The listing builds one solid part. Answer for the finished solid, in the listing's coordinates (mm). Face numbers are marked on the shaded views. Give positions to 0.01 mm unless a question says otherwise; leave off trailing zeros. Order: outer loops, then holes, each group sorted by start corner. A loop starts at its lowest first (then second) coordinate and runs counter-clockwise, first axis right, second up. Notation, with made-up numbers: (-12, -9.75) - (6, -9.75) arc R17 ccw to (6, 15.25) - close; hole circle Ø10 at (36.25, -2.5). An arc over 180 degrees is marked (long way). Answer as CSV lines item,"result". Start each with the question number.
1. Section C-C on y = 2.75 is taken. Give the vertices of the cut face in (x, z), and give its area (3 significant figures).
2. A flat-ended cylindrical pin translates along its axis: pin 1 (1.5 mm diameter, centred on x = 16.5, y = 12.5, fed in from -Z). Find the tip coordinate at first contact, or state that the pin passes through.
3. Section B-B on y = 22.5 is taken. Give the vertices of the cut face in (x, z).
4. Consider line 1 along X through (y, z) = (2.25, 8.25); line 2 along Y through (x, z) = (10, 4.75). Determine where each line is inside the solid, lowest interval first. Write a range as [from, to].
5. Determine the mould class of the marked faces 1, 2 and 3 for opening direction X: +X half, -X half, draft (parallel to the pull), parting line (faces both ways), or undercut.
6. Section A-A on z = 8.5 is taken. Give the vertices of the cut face in (x, y), and give its area (3 significant figures).
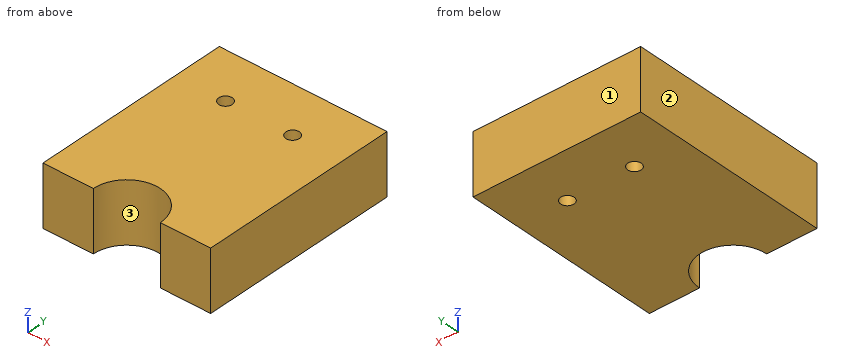
from build123d import *

# Parameters (mm, degrees)
SKETCH1_W           = 25
SKETCH1_H           = 30
BOSS_EXTRUDE1_DEPTH = 9
CUT_EXTRUDE3_DEPTH  = 41.074929819
SKETCH5_R           = 1
CUT_EXTRUDE4_DEPTH  = 41.074929819


with BuildPart() as part:
    # Sketch1 → Boss-Extrude1 (new body)
    with BuildSketch(Plane.XY):
        with Locations((12.5, 15)):
            Rectangle(SKETCH1_W, SKETCH1_H)
    extrude(amount=BOSS_EXTRUDE1_DEPTH)

    # Sketch4 → Cut-Extrude3 (cut, through all)
    with BuildSketch(Plane.XY.offset(9)):
        with BuildLine():
            ThreePointArc((17.5, 0), (12.5, 5), (7.5, 0))
            Line((7.5, 0), (17.5, 0))
        make_face()
        with BuildLine():
            Line((17.5, 0), (7.5, 0))
            ThreePointArc((7.5, 0), (12.5, -5), (17.5, 0))
        make_face()
    extrude(amount=-CUT_EXTRUDE3_DEPTH, mode=Mode.SUBTRACT)

    # Sketch5 → Cut-Extrude4 (cut, through all)
    with BuildSketch(Plane.XY.offset(9)):
        with Locations((7.5, 22.5)):
            Circle(SKETCH5_R)
        with Locations(Location((17.5, 22.5, 0), (0, 0, 180))):
            Circle(SKETCH5_R)
    extrude(amount=-CUT_EXTRUDE4_DEPTH, mode=Mode.SUBTRACT)


solid = part.part
Checks:
1,outline,"(0, 0) - (8.32, 0) - (8.32, 9) - (0, 9) - close; (16.68, 0) - (25, 0) - (25, 9) - (16.68, 9) - close"
1,area,"150 mm²"
2,pin 1,"stops at z = 0"
3,outline,"(0, 0) - (6.5, 0) - (6.5, 9) - (0, 9) - close; (8.5, 0) - (16.5, 0) - (16.5, 9) - (8.5, 9) - close; (18.5, 0) - (25, 0) - (25, 9) - (18.5, 9) - close"
4,line 1,"x = [0, 8.03], [16.97, 25]"
4,line 2,"y = [4.33, 30]"
5,face 1,"draft"
5,face 2,"-X half"
5,face 3,"undercut"
6,outline,"(0, 0) - (7.5, 0) arc R5 cw to (17.5, 0) - (25, 0) - (25, 30) - (0, 30) - close; hole circle Ø2 at (7.5, 22.5); hole circle Ø2 at (17.5, 22.5)"
6,area,"704 mm²"
